Autodesk Inventor part; units mm, degrees
ref_plane "YZ Plane" through (0, 0, 0) normal (1, 0, 0) x (0, 1, 0)
ref_plane "XZ Plane" through (0, 0, 0) normal (0, 1, 0) x (-1, 0, 0)
ref_plane "XY Plane" through (0, 0, 0) normal (0, 0, 1) x (1, 0, 0)
sketch "Sketch1" plane through (0, 0, 0) normal (0, 0, 1) x (1, 0, 0)
  circle A0 centre (0, 0) radius 5
  dimension "d0" = 10
extrude "Extrusion1" add sketch "Sketch1" along normal blind 6
sketch "Sketch2" plane through (0, 0, 6) normal (0, 0, 1) x (1, 0, 0)
  circle A0 centre (0, 0) radius 5
  circle A1 centre (0, 0) radius 3
  dimension "d3" = 6
extrude "Extrusion2" add sketch "Sketch2" along normal blind 25 contours A1
thread "Thread1"
chamfer "Chamfer1" distance 1 angle 45 1 edges at (-3, 0, 31)
chamfer "Chamfer2" distance 0.2 angle 45 1 edges at (-5, 0, 6)
fillet "Fillet1" radius 1 1 edges at (-5, 0, 0)
sketch "Sketch3" plane through (0, 0, 0) normal (0, 0, -1) x (-1, 0, 0)
  circle A0 centre (0, 0) radius 4
  line L0 (1.5588, 2.4297) -> (2.8836, -0.135)
  line L1 (2.8836, -0.135) -> (1.3248, -2.5648)
  line L2 (1.3248, -2.5648) -> (-1.5588, -2.4297)
  line L3 (-1.5588, -2.4297) -> (-2.8836, 0.135)
  line L4 (-2.8836, 0.135) -> (-1.3248, 2.5648)
  line L5 (-1.3248, 2.5648) -> (1.5588, 2.4297)
  dimension "d15" = 5
extrude "Extrusion3" cut sketch "Sketch3" against normal blind 5 contours L0 L1 L2 L3 L4 L5
sketch "Boceto4" plane through (0, 0, 31) normal (0, 0, 1) x (1, 0, 0)
  circle A0 centre (0, 0) radius 12.7903
extrude "Extrusión4" cut sketch "Boceto4" against normal blind 7.5
chamfer "Chaflán3" distance 1 angle 45 1 edges at (-3, 0, 23.5)
properties part number "PERNO PARKER M5"
Here's how the part is built. I have some questions about the finished solid (model axes, mm). A direction names the side the tool comes from. Give positions to 0.01 mm unless a question says otherwise; leave off trailing zeros. Order: outer loops, then holes, each group sorted by start corner. A loop starts at its lowest first (then second) coordinate and runs counter-clockwise, first axis right, second up. Notation, with made-up numbers: (-3.75, -29) - (0.25, -29) arc R23 cw to (0.25, -9) - close; hole circle Ø1 at (-1.75, 53.25). An arc over 180 degrees is marked (long way). Answer as a JSON object with one key per item and string values. Group by question number.
Item 1: If we section it at B-B on x = 0: Please give me the cut outline in (y, z).
Item 2: Please list where these lines run through material, in increasing order: probe 1 along X at (y, z) = (3, 2); probe 2 along Z at (x, y) = (4, -0.5).
Item 3: For P1, Ø1, axis at x = 3, y = 2, coming from the +Z side; P2, Ø4, axis at x = 0.5, z = 11, coming from the +Y side; P3, Ø1, axis at y = -1.5, z = 6, coming from the +X side, each with a flat end and sliding along its axis, tell me the tip position at first contact or that it passes through.
Item 4: If we mould it in two halves opening along Y, with no side actions, what happens to faces 4 (the flat face through (0, -3, 0)), 5 (the flat face through (0.1, -2.5, 2.5)), 6 (the cylindrical face through (-1.08, 4.88, 3.37))? For each: pulls with the +Y half, pulls with the -Y half, needs draft (parallel to the pull), parting line crosses it, or undercut.
Item 5: Which directions (+Z, -Z, +X, -X, +Y, -Y) give clear straight access to the entire face, cutting with the end or side of a thin tool? Please do faces 1 (the flat face through (1, -3, 6)), 2 (the flat face through (0, 0, 5)), 3 (the flat face through (0, 0, 23.5)).
Item 6: If we section it at C-C on z = 7.5: Please give me the cut outline in (x, y).
Item 7: If we section it at A-A on z = 3.75: Please give me the cut outline in (x, y) (3 decimals), and give its area (3 significant figures).
Result set:
{
 "1": {"outline": "(-5, 1) arc R1 ccw to (-4, 0) - (-2.5, 0) - (-2.5, 5) - (2.5, 5) - (2.5, 0) - (4, 0) arc R1 ccw to (5, 1) - (5, 5.8) - (4.8, 6) - (3, 6) - (3, 22.5) - (2, 23.5) - (-2, 23.5) - (-3, 22.5) - (-3, 6) - (-4.8, 6) - (-5, 5.8) - close"},
 "2": {"probe 1": "-4 to 4", "probe 2": "0 to 6"},
 "3": {"P1": "z = 6", "P2": "y = 3", "P3": "x = 4.89"},
 "4": {"face 4": "needs draft", "face 5": "undercut", "face 6": "parting line crosses it"},
 "5": {"face 1": "+Z", "face 2": "-Z", "face 3": "+Z, +X, -X, +Y, -Y"},
 "6": {"outline": "circle Ø6 at (0, 0)"},
 "7": {"outline": "circle Ø10 at (0, 0); hole (-2.884, -0.135) - (-1.325, -2.565) - (1.559, -2.43) - (2.884, 0.135) - (1.325, 2.565) - (-1.559, 2.43) - close", "area": "56.9 mm²"}
}
